Design review of the part built by this model. Coordinates are the model's own, in mm. Round coordinates to 2 decimals unless told otherwise and drop trailing zeros. Loops run counter-clockwise (first coordinate to the right, second up) from the corner with the lowest first, then second, coordinate; pieces in that order, holes last. Notation, with made-up numbers: (10, 9) - (42, 9) arc R28 ccw to (42, 45) - close; hole circle Ø10 at (18.25, 65.5). An arc over 180 degrees is marked (long way). Use one line per item in the form item = value. Start each with the question number.
(1) We need section B-B, the plane y = -205.5. Write out the cut boundary in (x, z), then the cut area to 3 significant figures.
(2) For pin 1 (1 mm diameter, centred on x = -204, z = 25, fed in from -Y), flat-tipped, find the tip position at first contact; note if it passes through.
(3) We need section A-A, the plane z = 31. Write out the cut boundary in (x, y), then the cut area to 3 significant figures.
(4) Wall thickness on probe 1 along X at (y, z) = (-572, 15.5); probe 2 along Y at (x, z) = (257, 21): over which ranges is each line inside the solid? List them lowest first. Write a range as [from, to].
(5) We need section C-C, the plane x = -127.5. Write out the cut boundary in (y, z), then the cut area to 3 significant figures.
from build123d import *

# Parameters (mm, degrees)
F1_DEPTH = 38.1


with BuildPart() as f1:
    # F0 (on Top) → F1 (new body)
    with BuildSketch(Plane.XY):
        with BuildLine():
            Line((368.3, 679.45), (-368.3, 679.45))
            ThreePointArc((-368.3, 679.45), (-404.221024, 664.571024), (-419.1, 628.65))
            Line((-419.1, 628.65), (-419.1, -679.45))
            Line((-419.1, -679.45), (-381, -679.45))
            Line((-381, -679.45), (-381, 133.35))
            Line((-381, 133.35), (381, 133.35))
            Line((381, 133.35), (381, -679.45))
            Line((381, -679.45), (419.1, -679.45))
            Line((419.1, -679.45), (419.1, 628.65))
            ThreePointArc((419.1, 628.65), (404.221024, 664.571024), (368.3, 679.45))
        make_face()
    extrude(amount=F1_DEPTH)


solid = f1.part
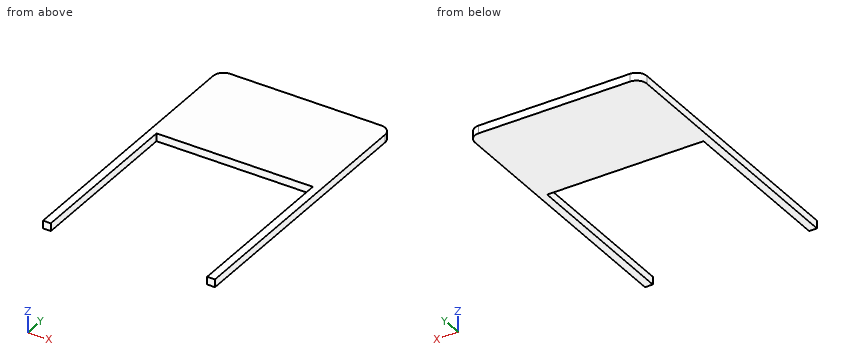
Data:
q1.outline = (-419.1, 0) - (-381, 0) - (-381, 38.1) - (-419.1, 38.1) - close; (381, 0) - (419.1, 0) - (419.1, 38.1) - (381, 38.1) - close
q1.area = 2,900 mm^2
q2.pin_1 = 133.35
q3.outline = (-419.1, -679.45) - (-381, -679.45) - (-381, 133.35) - (381, 133.35) - (381, -679.45) - (419.1, -679.45) - (419.1, 628.65) arc R50.8 ccw to (368.3, 679.45) - (-368.3, 679.45) arc R50.8 ccw to (-419.1, 628.65) - close
q3.area = 519,000 mm^2
q4.probe_1 = [-419.1, -381], [381, 419.1]
q4.probe_2 = [133.35, 679.45]
q5.outline = (133.35, 0) - (679.45, 0) - (679.45, 38.1) - (133.35, 38.1) - close
q5.area = 20,800 mm^2
